Answer from the drawing. Dimensions are ordinates in mm from the lowest x, y and z of the part. A direction names the side the tool comes from. Coordinates: 2 decimals unless noted, no trailing zeros. Write each loop counter-clockwise with the first axis right and the second up, starting at its lowest first coordinate (ties: lowest second). Pieces come first, ordered by that corner, then holes. Notation, with made-up numbers: (7.5, 74) -> (11.5, 74) arc R31 cw to (11.5, 113) -> close; hole circle Ø11 at (-2.75, 61). An arc over 180 degrees is marked (long way). Use CSV: the item, a comma, the result in double quotes.
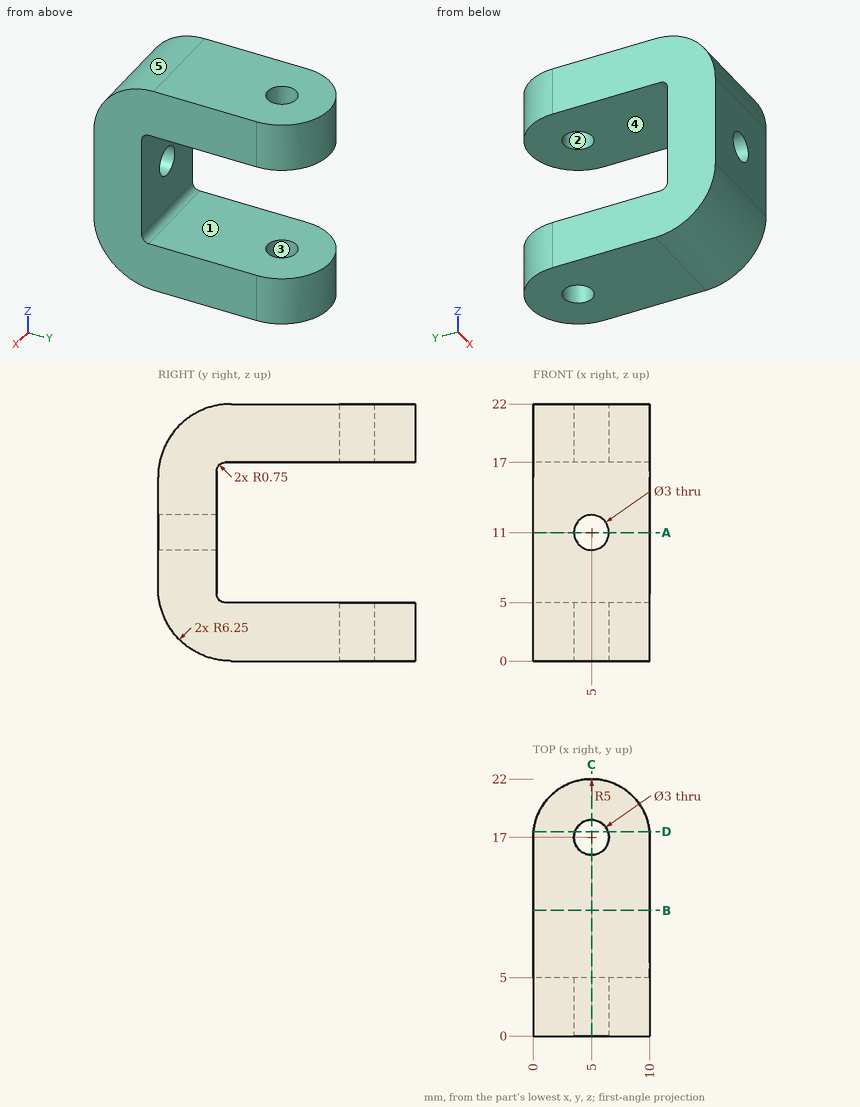
1. This flat-tipped pin is pushed along its axis until it touches: pin 1 Ø5 at (x, z) = (5, 11) entering from +Y. Where does it stop, or does it pass through?
Solutions:
pin 1,"stops at y = 5"
2. A cutting plane is placed at B-B (y = 10.75). Give the vertices of the cut face in (x, z), and give its area (3 significant figures).
Solutions:
outline,"(0, 0) -> (10, 0) -> (10, 5) -> (0, 5) -> close; (0, 17) -> (10, 17) -> (10, 22) -> (0, 22) -> close"
area,"100 mm^2"
3. A cutting plane is placed at A-A (z = 11). Give the vertices of the cut face in (x, y).
Solutions:
outline,"(0, 0) -> (3.5, 0) -> (3.5, 5) -> (0, 5) -> close; (6.5, 0) -> (10, 0) -> (10, 5) -> (6.5, 5) -> close"
4. For a pull along Z with two mould halves and no side action, classify the marked faces 3, 4 and 5 as pulls with the +Z half, pulls with the -Z half, needs draft (parallel to the pull), parting line crosses it, or undercut.
Solutions:
face 3,"needs draft"
face 4,"undercut"
face 5,"pulls with the +Z half"
5. A cutting plane is placed at C-C (x = 5). Give the vertices of the cut face in (y, z), and give its area (3 significant figures).
Solutions:
outline,"(0, 6.25) arc R6.25 ccw to (6.25, 0) -> (15.5, 0) -> (15.5, 5) -> (5.75, 5) arc R0.75 cw to (5, 5.75) -> (5, 9.5) -> (0, 9.5) -> close; (0, 12.5) -> (5, 12.5) -> (5, 16.25) arc R0.75 cw to (5.75, 17) -> (15.5, 17) -> (15.5, 22) -> (6.25, 22) arc R6.25 ccw to (0, 15.75) -> close; (18.5, 0) -> (22, 0) -> (22, 5) -> (18.5, 5) -> close; (18.5, 17) -> (22, 17) -> (22, 22) -> (18.5, 22) -> close"
area,"218 mm^2"
6. Find the intervals of material crossed by line 1 along X through (y, z) = (17, 20.75); line 2 along Z through (x, y) = (3, 20.25); line 3 along Y through (x, z) = (1.5, 10), in increasing order.
Solutions:
line 1,"x = 0 to 3.5, 6.5 to 10"
line 2,"z = 0 to 5, 17 to 22"
line 3,"y = 0 to 5"
7. A tool of negligible diameter and unlimited length cuts with its end or side. For the marked faces 1 and 2, from which of +Z, -Z, +X, -X, +Y, -Y can it reach the whole face along a straight path? Write none if from no direction.
Solutions:
face 1,"+X, -X, +Y"
face 2,"+Z, -Z"
8. A cutting plane is placed at D-D (y = 17.5). Give the vertices of the cut face in (x, z).
Solutions:
outline,"(0.03, 0) -> (3.59, 0) -> (3.59, 5) -> (0.03, 5) -> close; (0.03, 17) -> (3.59, 17) -> (3.59, 22) -> (0.03, 22) -> close; (6.41, 0) -> (9.97, 0) -> (9.97, 5) -> (6.41, 5) -> close; (6.41, 17) -> (9.97, 17) -> (9.97, 22) -> (6.41, 22) -> close"
